Part model, mm, in its own coordinate system. A direction names the side the tool comes from. Coordinates: 2 decimals unless noted, no trailing zeros. Write each loop counter-clockwise with the first axis right and the second up, starting at its lowest first coordinate (ties: lowest second). Pieces come first, ordered by that corner, then holes. Notation, with made-up numbers: (-28.5, 82.5) - (-19.5, 82.5) arc R17 ccw to (-19.5, 110.5) - close; hole circle Ø3 at (46, 8.25). An arc over 180 degrees is marked (long way). Write each question's results on one line, items separated by ' | '.
from build123d import *

# Parameters (mm, degrees)
SKETCH_1_W          = 45
SKETCH_1_H          = 10
EXTRUDE_1_DEPTH     = 5
SKETCH_2_W          = 5
SKETCH_2_H          = 4
EXTRUDE_2_DEPTH     = 11
SKETCH_3_W          = 5
SKETCH_3_H          = 2
CUT_EXTRUDE_1_DEPTH = 3
SKETCH_4_W          = 5
SKETCH_4_H          = 2
CUT_EXTRUDE_2_DEPTH = 3
SKETCH_7_W          = 5
SKETCH_7_H          = 4
EXTRUDE_3_DEPTH     = 11
SKETCH_8_W          = 5
SKETCH_8_H          = 2
CUT_EXTRUDE_5_DEPTH = 3
SKETCH_9_W          = 5
SKETCH_9_H          = 2
CUT_EXTRUDE_6_DEPTH = 3


with BuildPart() as part:
    # Эскиз1 → Бобышка-Вытянуть1 (new body)
    with BuildSketch(Plane.XY):
        Rectangle(SKETCH_1_W, SKETCH_1_H)
    extrude(amount=EXTRUDE_1_DEPTH)

    # Эскиз2 → Бобышка-Вытянуть2 (add)
    with BuildSketch(Plane.XY.offset(5)):
        with Locations((-10, 3)):
            Rectangle(SKETCH_2_W, SKETCH_2_H)
        with Locations((10, 3)):
            Rectangle(SKETCH_2_W, SKETCH_2_H)
    extrude(amount=EXTRUDE_2_DEPTH)

    # Эскиз3 → Вырез-Вытянуть1 (cut)
    with BuildSketch(Plane.XY.offset(16)):
        with Locations((-10, 2)):
            Rectangle(SKETCH_3_W, SKETCH_3_H)
    extrude(amount=-CUT_EXTRUDE_1_DEPTH, mode=Mode.SUBTRACT)

    # Эскиз4 → Вырез-Вытянуть2 (cut)
    with BuildSketch(Plane.XY.offset(16)):
        with Locations((10, 2)):
            Rectangle(SKETCH_4_W, SKETCH_4_H)
    extrude(amount=-CUT_EXTRUDE_2_DEPTH, mode=Mode.SUBTRACT)

    # Эскиз7 → Бобышка-Вытянуть3 (add)
    with BuildSketch(Plane.XY.offset(5)):
        with Locations((-10, -3)):
            Rectangle(SKETCH_7_W, SKETCH_7_H)
        with Locations((10, -3)):
            Rectangle(SKETCH_7_W, SKETCH_7_H)
    extrude(amount=EXTRUDE_3_DEPTH)

    # Эскиз8 → Вырез-Вытянуть5 (cut)
    with BuildSketch(Plane.XY.offset(16)):
        with Locations((-10, -2)):
            Rectangle(SKETCH_8_W, SKETCH_8_H)
    extrude(amount=-CUT_EXTRUDE_5_DEPTH, mode=Mode.SUBTRACT)

    # Эскиз9 → Вырез-Вытянуть6 (cut)
    with BuildSketch(Plane.XY.offset(16)):
        with Locations((10, -2)):
            Rectangle(SKETCH_9_W, SKETCH_9_H)
    extrude(amount=-CUT_EXTRUDE_6_DEPTH, mode=Mode.SUBTRACT)


solid = part.part
(1) Wall check: line 1 (Y direction, x = -10.5, z = 5.25); line 2 (X direction, y = 2.5, z = 5.5); line 3 (Z direction, x = 2, y = -3.75). Give the ranges that are in metal, low to high. Write a range as from..to.
Return value:
line 1: y = -5..-1, 1..5 | line 2: x = -12.5..-7.5, 7.5..12.5 | line 3: z = 0..5
(2) Saw through at A-A on z = 14.75. Write the cut outline in (x, y).
Return value:
outline: (-12.5, -5) - (-7.5, -5) - (-7.5, -3) - (-12.5, -3) - close; (-12.5, 3) - (-7.5, 3) - (-7.5, 5) - (-12.5, 5) - close; (7.5, -5) - (12.5, -5) - (12.5, -3) - (7.5, -3) - close; (7.5, 3) - (12.5, 3) - (12.5, 5) - (7.5, 5) - close
(3) Saw through at C-C on z = 12.5. Write the cut outline in (x, y), then the cut area to 3 significant figures.
Return value:
outline: (-12.5, -5) - (-7.5, -5) - (-7.5, -1) - (-12.5, -1) - close; (-12.5, 1) - (-7.5, 1) - (-7.5, 5) - (-12.5, 5) - close; (7.5, -5) - (12.5, -5) - (12.5, -1) - (7.5, -1) - close; (7.5, 1) - (12.5, 1) - (12.5, 5) - (7.5, 5) - close | area: 80.0 mm^2
(4) Saw through at D-D on y = 4. Write the cut outline in (x, z), then the cut area to 3 significant figures.
Return value:
outline: (-22.5, 0) - (22.5, 0) - (22.5, 5) - (12.5, 5) - (12.5, 16) - (7.5, 16) - (7.5, 5) - (-7.5, 5) - (-7.5, 16) - (-12.5, 16) - (-12.5, 5) - (-22.5, 5) - close | area: 335 mm^2
(5) 3-axis set-ups, long thin cutter, end or side, ignore diameter. For faces 1 (the flat face through (-12.5, 3, 10)), 2 (the flat face through (-7.5, -3, 10)), 3 (the flat face through (12.5, -3, 10)), 4 (the flat face through (-10, -2, 13)): which of +Z, -Z, +X, -X, +Y, -Y reach the whole face in a straight line?
Return value:
face 1: +Z, -X, +Y, -Y | face 2: +Z, +Y, -Y | face 3: +Z, +X, +Y, -Y | face 4: +Z, +X, -X
(6) Two-plate mould, pull along Y, no slides. Class faces 5 (the flat face through (7.5, 3, 10)), 6 (the flat face through (0, 5, 4)), 7 (the flat face through (10, 2, 13)): released by +Y, released by -Y, zero draft, split by the parting line, or undercut.
Return value:
face 5: zero draft | face 6: released by +Y | face 7: undercut
(7) Saw through at B-B on y = 1.5. Write the cut outline in (x, z), then the cut area to 3 significant figures.
Return value:
outline: (-22.5, 0) - (22.5, 0) - (22.5, 5) - (12.5, 5) - (12.5, 13) - (7.5, 13) - (7.5, 5) - (-7.5, 5) - (-7.5, 13) - (-12.5, 13) - (-12.5, 5) - (-22.5, 5) - close | area: 305 mm^2
(8) Flat gauge pins, fed straight in: P1, Ø2, axis at x = 5.5, z = 13, coming from the -Y side; P2, Ø2, axis at y = 2.5, z = 8, coming from the +X side; P3, Ø4.5, axis at y = -3.5, z = 9, coming from the -X side; P4, Ø1.6, axis at x = 10, y = -2, coming from the +Z side. Where does each tip first touch, or does it go through?
Return value:
P1: passes through | P2: stops at x = 12.5 | P3: stops at x = -12.5 | P4: stops at z = 13
